Could you check a few things on this model? Use its own coordinates, in mm. A direction names the side the tool comes from. Round coordinates to 2 decimals unless told otherwise and drop trailing zeros. Answer as CSV lines item,"result". Start each with the question number.
1) I'm going to push flat-ended pins straight in: pin 1 Ø0.6 at (x, y) = (35.5, 5) entering from +Z; pin 2 Ø6 at (x, z) = (-13, -3) entering from -Y; pin 3 Ø6 at (x, z) = (37, -1.5) entering from -Y. Where does each tip first touch, or does it pass through?
2) Please list where these lines run through material, in increasing order: line 1 along Z through (x, y) = (-31, 3.5); line 2 along Z through (x, y) = (-36, 7.25); line 3 along Y through (x, z) = (24, -1).
3) Suppose I cut it at B-B, the plane y = 8.5. Count the separate pieces of the cut face and the enclosed holes in it, then the cut area to 3 significant figures.
4) Which directions (+Z, -Z, +X, -X, +Y, -Y) give clear straight access to the entire face, cutting with the end or side of a thin tool? Please do faces 1 (the face through (-47.49, 10.15, -0.07)), 2 (the face through (-1, 9, 13)).
5) We'd pull the mould along Z, two halves only. Please class faces 3 (the face through (-0.52, 0.86, 17.1)), 4 (the face through (37, 6, 0)), 5 (the face through (0.52, 10.15, -14.99)): pulls with the +Z half, pulls with the -Z half, needs draft (parallel to the pull), parting line crosses it, or undercut.
```python
from build123d import *

# Parameters (mm, degrees)
EXTRUDE_1_DEPTH = 10
SHELL_2_T       = 3
FILLET_3_R      = 10
FILLET_4_R      = 3
SKETCH_2_R      = 2.675
EXTRUDE_2_DEPTH = 8
EXTRUDE_3_DEPTH = 4
FILLET_11_R     = 0.3
FILLET_7_R      = 5
CHAMFER_1_SIZE  = 0.2
CHAMFER_2_SIZE  = 0.2
FILLET_9_SIZE   = 5.5
FILLET_9_SIZE_2 = 5


# Some blends are built 0.0001 mm under size
with BuildPart() as part:
    # 草图1 → 凸台-拉伸1 (new body)
    with BuildSketch(Plane(origin=(0, 0, 0), x_dir=(1, 0, 0), z_dir=(0, 1, 0))):
        with BuildLine():
            Line((-37.5, 15), (37.5, 15))
            ThreePointArc((37.5, 15), (44.571067812, 12.071067812), (47.5, 5))
            Line((47.5, 5), (47.5, -5))
            ThreePointArc((47.5, -5), (44.571067812, -12.071067812), (37.5, -15))
            Line((37.5, -15), (-37.5, -15))
            ThreePointArc((-37.5, -15), (-44.571067812, -12.071067812), (-47.5, -5))
            Line((-47.5, -5), (-47.5, 5))
            ThreePointArc((-47.5, 5), (-44.571067812, 12.071067812), (-37.5, 15))
        make_face()
    extrude(amount=EXTRUDE_1_DEPTH)

    # 抽壳2
    shell_2_openings = [part.faces().sort_by_distance(p)[0] for p in [
        (0, 0, 0),
    ]]
    offset(amount=SHELL_2_T, openings=shell_2_openings, kind=Kind.INTERSECTION)

    # 圆角3
    # the kernel refuses this fillet: 10 mm, written as the material it takes off along each edge
    with BuildSketch(Plane(origin=(37.5, 13, 5), x_dir=(1, 0, 0), z_dir=(0, 0, -1))) as fillet_3_piece_1:
        with BuildLine():
            CenterArc((13 - FILLET_3_R, FILLET_3_R), FILLET_3_R, 270, 90)
            Line((13 - FILLET_3_R, 0), (13, 0))
            Line((13, 0), (13, FILLET_3_R))
        make_face()
    revolve(axis=Axis((37.5, 13, 5), (0, -1, 0)), revolution_arc=90, mode=Mode.SUBTRACT)
    with BuildSketch(Plane(origin=(50.5, 13, 5), x_dir=(0, -1, 0), z_dir=(0, 0, -1)), Plane(origin=(-50.5, 13, -5), x_dir=(0, -1, 0), z_dir=(0, 0, 1))) as fillet_3_piece_2:
        with BuildLine():
            CenterArc((FILLET_3_R, FILLET_3_R), FILLET_3_R, 180, 90)
            Line((0, FILLET_3_R), (0, 0))
            Line((0, 0), (FILLET_3_R, 0))
        make_face()
    extrude(amount=10, mode=Mode.SUBTRACT)
    with BuildSketch(Plane(origin=(37.5, 13, -5), x_dir=(0, 0, -1), z_dir=(-1, 0, 0))) as fillet_3_piece_3:
        with BuildLine():
            CenterArc((13 - FILLET_3_R, FILLET_3_R), FILLET_3_R, 270, 90)
            Line((13 - FILLET_3_R, 0), (13, 0))
            Line((13, 0), (13, FILLET_3_R))
        make_face()
    revolve(axis=Axis((37.5, 13, -5), (0, -1, 0)), revolution_arc=90, mode=Mode.SUBTRACT)
    with BuildSketch(Plane(origin=(37.5, 13, -18), x_dir=(0, -1, 0), z_dir=(-1, 0, 0)), Plane(origin=(-37.5, 13, 18), x_dir=(0, -1, 0), z_dir=(1, 0, 0))) as fillet_3_piece_4:
        with BuildLine():
            CenterArc((FILLET_3_R, FILLET_3_R), FILLET_3_R, 180, 90)
            Line((0, FILLET_3_R), (0, 0))
            Line((0, 0), (FILLET_3_R, 0))
        make_face()
    extrude(amount=75, mode=Mode.SUBTRACT)
    with BuildSketch(Plane(origin=(-37.5, 13, -5), x_dir=(-1, 0, 0), z_dir=(0, 0, 1))) as fillet_3_piece_5:
        with BuildLine():
            CenterArc((13 - FILLET_3_R, FILLET_3_R), FILLET_3_R, 270, 90)
            Line((13 - FILLET_3_R, 0), (13, 0))
            Line((13, 0), (13, FILLET_3_R))
        make_face()
    revolve(axis=Axis((-37.5, 13, -5), (0, -1, 0)), revolution_arc=90, mode=Mode.SUBTRACT)
    with BuildSketch(Plane(origin=(-37.5, 13, 5), x_dir=(0, 0, 1), z_dir=(1, 0, 0))) as fillet_3_piece_6:
        with BuildLine():
            CenterArc((13 - FILLET_3_R, FILLET_3_R), FILLET_3_R, 270, 90)
            Line((13 - FILLET_3_R, 0), (13, 0))
            Line((13, 0), (13, FILLET_3_R))
        make_face()
    revolve(axis=Axis((-37.5, 13, 5), (0, -1, 0)), revolution_arc=90, mode=Mode.SUBTRACT)

    # 圆角4
    fillet_4_edges = [part.edges().sort_by_distance(p)[0] for p in [
        (50.5, 0, 0),
        (46.692388155, 0, 14.192388155),
        (0, 0, 18),
        (-46.692388155, 0, 14.192388155),
        (-50.5, 0, 0),
        (-46.692388155, 0, -14.192388155),
        (0, 0, -18),
        (46.692388155, 0, -14.192388155),
    ]]
    fillet(fillet_4_edges, radius=FILLET_4_R - 0.0001)  # a hair under: the kernel refuses the full size

    # 草图2 → 凸台-拉伸2 (add)
    # profile 1 of 2: a face of its own
    with BuildSketch(Plane(origin=(0, 10, 0), x_dir=(-1, 0, 0), z_dir=(0, -1, 0))):
        with Locations(Location((36.8, 0, 0), (0, 0, 270))):
            Circle(SKETCH_2_R)
        Polygon((34.725, -0.575), (34.725, 0.575), (36.225, 0.575), (36.225, 2.075), (37.375, 2.075), (37.375, 0.575), (38.875, 0.575), (38.875, -0.575), (37.375, -0.575), (37.375, -2.075), (36.225, -2.075), (36.225, -0.575), align=None, mode=Mode.SUBTRACT)
    # profile 2 of 2: a face of its own
    with BuildSketch(Plane(origin=(0, 10, 0), x_dir=(-1, 0, 0), z_dir=(0, -1, 0))):
        with Locations(Location((-36.8, 0, 0), (0, 0, 90))):
            Circle(SKETCH_2_R)
        Polygon((-37.375, 0.575), (-37.375, 2.075), (-36.225, 2.075), (-36.225, 0.575), (-34.725, 0.575), (-34.725, -0.575), (-36.225, -0.575), (-36.225, -2.075), (-37.375, -2.075), (-37.375, -0.575), (-38.875, -0.575), (-38.875, 0.575), align=None, mode=Mode.SUBTRACT)
    extrude(amount=EXTRUDE_2_DEPTH)

    # 草图3 → 凸台-拉伸3 (add)
    with BuildSketch(Plane.XZ.offset(-10)):
        Polygon((-37.375, -2.075), (-36.225, -2.075), (-36.225, -0.575), (-34.725, -0.575), (-34.725, 0.575), (-36.225, 0.575), (-36.225, 2.075), (-37.375, 2.075), (-37.375, 0.575), (-38.875, 0.575), (-38.875, -0.575), (-37.375, -0.575), align=None)
        Polygon((34.725, 0.575), (34.725, -0.575), (36.225, -0.575), (36.225, -2.075), (37.375, -2.075), (37.375, -0.575), (38.875, -0.575), (38.875, 0.575), (37.375, 0.575), (37.375, 2.075), (36.225, 2.075), (36.225, 0.575), align=None)
    extrude(amount=EXTRUDE_3_DEPTH)

    # 圆角11
    fillet_11_edges = [part.edges().sort_by_distance(p)[0] for p in [
        (36.225, 4, -0.575),
        (36.225, 4, 0.575),
        (37.375, 4, 0.575),
        (37.375, 4, -0.575),
        (-37.375, 4, -0.575),
        (-37.375, 4, 0.575),
        (-36.225, 4, 0.575),
        (-36.225, 4, -0.575),
    ]]
    fillet(fillet_11_edges, radius=FILLET_11_R)

    # 圆角7
    fillet_7_edges = [part.edges().sort_by_distance(p)[0] for p in [
        (-44.571067812, 10, 12.071067812),
        (0, 10, 15),
        (44.571067812, 10, 12.071067812),
        (47.5, 10, 0),
        (44.571067812, 10, -12.071067812),
        (0, 10, -15),
        (-44.571067812, 10, -12.071067812),
        (-47.5, 10, 0),
    ]]
    fillet(fillet_7_edges, radius=FILLET_7_R)

    # 倒角1
    chamfer_1_edges = [part.edges().sort_by_distance(p)[0] for p in [
        (35.325, 2, -0.575),
        (38.875, 2, 0),
        (37.375, 2, -1.475),
        (36.8, 2, -2.075),
        (34.725, 2, 0),
        (35.325, 2, 0.575),
        (36.8, 2, 2.075),
        (36.225, 2, -1.475),
        (38.275, 2, -0.575),
        (36.225, 2, 1.475),
        (37.375, 2, 1.475),
        (38.275, 2, 0.575),
        (37.462867966, 2, 0.662867966),
        (36.137132034, 2, 0.662867966),
        (36.137132034, 2, -0.662867966),
        (37.462867966, 2, -0.662867966),
    ]]
    chamfer(chamfer_1_edges, length=CHAMFER_1_SIZE)

    # 倒角2
    chamfer_2_edges = [part.edges().sort_by_distance(p)[0] for p in [
        (-36.8, 2, -2.075),
        (-37.375, 2, -1.475),
        (-38.875, 2, 0),
        (-35.325, 2, -0.575),
        (-38.275, 2, -0.575),
        (-38.275, 2, 0.575),
        (-37.375, 2, 1.475),
        (-36.225, 2, 1.475),
        (-37.462867966, 2, 0.662867966),
        (-36.137132034, 2, 0.662867966),
        (-36.137132034, 2, -0.662867966),
        (-37.462867966, 2, -0.662867966),
        (-36.8, 2, 2.075),
        (-35.325, 2, 0.575),
        (-34.725, 2, 0),
        (-36.225, 2, -1.475),
    ]]
    chamfer(chamfer_2_edges, length=CHAMFER_2_SIZE)

    # 圆角9
    # a fillet whose section is not a circle: 5.5, 5 mm, written as the material it adds along each edge
    with BuildSketch(Plane(origin=(36.8, 10, 0), x_dir=(0, 0, -1), z_dir=(-1, 0, 0))) as fillet_9_piece_1:
        with BuildLine():
            Bezier((2.675 + FILLET_9_SIZE, 0), (2.675, 0), (2.675, FILLET_9_SIZE_2), weights=[1, 0.333333333, 1])
            Line((2.675, FILLET_9_SIZE_2), (2.675, 0))
            Line((2.675, 0), (2.675 + FILLET_9_SIZE, 0))
        make_face()
    revolve(axis=Axis((36.8, 10, 0), (0, -1, 0)))

    # 圆角10
    # a fillet whose section is not a circle: 5.5, 5 mm, written as the material it adds along each edge (its section moved 0.00015 mm through the faces so that the kernel can cut it)
    with BuildSketch(Plane(origin=(-36.8, 10, 0), x_dir=(0, 0, 1), z_dir=(1, 0, 0))) as fillet_10_piece_1:
        with BuildLine():
            Bezier((7.675, -0.00015), (2.67485, -0.00015), (2.67485, 5.5), weights=[1, 0.333333333, 1])
            Line((2.67485, 5.5), (2.56485, 5.5))
            ThreePointArc((2.56485, 5.5), (2.565, 2.75), (2.565, 0))
            Line((2.565, 0), (2.675, -0.11))
            ThreePointArc((2.675, -0.11), (5.175, -0.11), (7.675, -0.11015))
            Line((7.675, -0.11015), (7.675, -0.00015))
        make_face()
    revolve(axis=Axis((-36.8, 10, 0), (0, -1, 0)))


solid = part.part
```
Filled sheet:
1,pin 1,"z = 17.85"
1,pin 2,"y = 10"
1,pin 3,"y = 2"
2,line 1,"-17.99 to -15, 15 to 17.99"
2,line 2,"-17.05 to -14.47, -3.89 to 3.89, 14.47 to 17.05"
2,line 3,"10 to 13"
3,separate pieces,"3"
3,enclosed holes,"1"
3,area,"813 mm²"
4,face 1,"+Z, -Z, -X, +Y"
4,face 2,"-Y"
5,face 3,"pulls with the +Z half"
5,face 4,"undercut"
5,face 5,"pulls with the -Z half"
